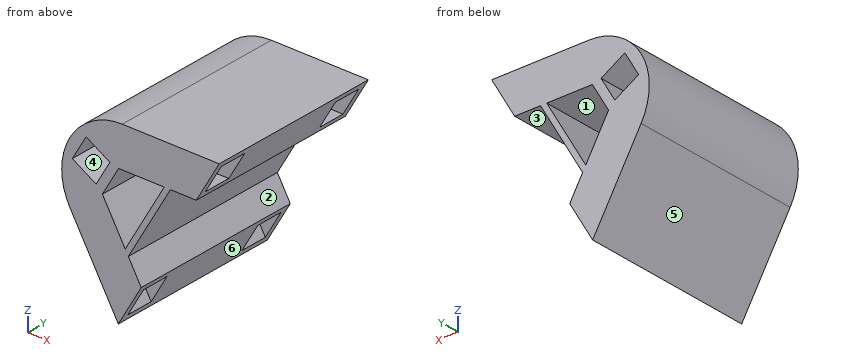
from build123d import *

# Parameters (mm, degrees)
BOSS_EXTRUDE1_DEPTH     = 130
SKETCH2_W               = 100.4
SKETCH2_H               = 20.4
CUT_EXTRUDE2_DEPTH      = 20.4
CUT_EXTRUDE3_DEPTH      = 238.223523286
FILLET1_R               = 45
CUT_EXTRUDE4_DEPTH      = 238.223523286
CUT_EXTRUDE4_DEPTH_BACK = 238.223523286
BOSS_EXTRUDE2_DEPTH     = 130


with BuildPart() as part:
    # Sketch1 → Boss-Extrude1 (new body)
    with BuildSketch(Plane(origin=(0, 0, 0), x_dir=(1, 0, 0), z_dir=(0, 1, 0))):
        Polygon((0, 0), (150, 0), (75, 129.903810568), align=None)
    extrude(amount=BOSS_EXTRUDE1_DEPTH)

    # Sketch2 → Cut-Extrude2 (cut)
    with BuildSketch(Plane(origin=(0, 5, 0), x_dir=(1, 0, 0), z_dir=(0, 1, 0))):
        Polygon((108.923840175, 138.261625339), (58.723840175, 51.312674799), (41.056921938, 61.512674799), (91.256921938, 148.461625339), align=None)
        with Locations((124, 15)):
            Rectangle(SKETCH2_W, SKETCH2_H)
    cut_extrude2 = extrude(amount=CUT_EXTRUDE2_DEPTH, mode=Mode.SUBTRACT)

    # Mirror1: Cut-Extrude2 across plane
    add(cut_extrude2.mirror(Plane.ZX.offset(65)), mode=Mode.SUBTRACT)

    # Sketch4 → Cut-Extrude3 (cut, through all)
    with BuildSketch(Plane(origin=(0, 0, 0), x_dir=(1, 0, 0), z_dir=(0, 1, 0))):
        Polygon((58.515583945, 45.561933634), (40.848665708, 35.361933634), (51.048665708, 17.695015397), (68.715583945, 27.895015397), align=None)
    extrude(amount=CUT_EXTRUDE3_DEPTH, mode=Mode.SUBTRACT)

    # Fillet1
    fillet1_edges = [part.edges().sort_by_distance(p)[0] for p in [
        (0, 65, 0),
    ]]
    fillet(fillet1_edges, radius=FILLET1_R)

    # Sketch27 → Cut-Extrude4 (cut, two sides: drawn at the far end of the back side and taken through both)
    with BuildSketch(Plane.XZ.offset(-CUT_EXTRUDE4_DEPTH_BACK)):
        Polygon((426.334426918, -29.530127019), (132.950773216, -29.530127019), (75.215746297, -29.530127019), (63.181713324, -50.373683549), (92.049226784, -100.373683549), (238.741053634, -354.45138071), (746.896447956, -647.835034411), (934.48982124, -322.913780721), align=None)
    extrude(amount=CUT_EXTRUDE4_DEPTH + CUT_EXTRUDE4_DEPTH_BACK, mode=Mode.SUBTRACT)

    # Sketch28 → Boss-Extrude2 (add)
    with BuildSketch(Plane.XZ):
        Polygon((109.106207099, -29.530127019), (80.126943725, -79.723683549), (82.436344802, -83.723683549), (113.725009252, -29.530127019), align=None)
    extrude(amount=-BOSS_EXTRUDE2_DEPTH)


solid = part.part
Can you work these out from the model? Positions are in its coordinate system, mm. Face numbers are marked on the shaded views. A direction names the side the tool comes from. Give positions to 0.01 mm unless a question says otherwise; leave off trailing zeros. Loops run counter-clockwise (first coordinate to the right, second up) from the corner with the lowest first, then second, coordinate; pieces in that order, holes last. Notation, with made-up numbers: (36.25, 54) -> (95.25, 54) arc R20 cw to (95.25, 65) -> close; hole circle Ø9 at (21, 10). An arc over 180 degrees is marked (long way). Use one line per item in the form item = value.
1) If we section it at C-C (z = -41): Please give me the cut outline in (x, y).
Answers:
outline = (33.12, 0) -> (50.61, 0) -> (50.61, 130) -> (33.12, 130) -> close; (61.15, 0) -> (68.59, 0) -> (68.59, 130) -> (61.15, 130) -> close; (102.48, 0) -> (107.1, 0) -> (107.1, 130) -> (102.48, 130) -> close
2) I need wall thicknesses on line 1 along Y through (x, z) = (122, -8.5); line 2 along Z through (x, y) = (92, 53); line 3 along Z through (x, y) = (83, 17.5). Which ranges of each line are inside material? Lowest first, please.
Answers:
line_1 = 0 to 5, 25.4 to 104.6, 125 to 130
line_2 = -100.46 to -100.29, -67.16 to -59.16, -29.53 to 0
line_3 = -93.36 to -84.7, -82.75 to -74.75, -29.53 to -25.2, -4.8 to 0
3) We'd pull the mould along X, two halves only. Please class the marked faces 4, 5 and 6: released by +X, released by -X, zero draft, split by the parting line, or undercut.
Answers:
face_4 = undercut
face_5 = released by -X
face_6 = released by +X
4) For the marked faces 1, 2 and 3, which set-ups out of +Z, -Z, +X, -X, +Y, -Y let a thin tool reach every point of the face, with its end or its side?
Answers:
face_1 = +Y, -Y
face_2 = +X, +Y, -Y
face_3 = -Z, +X, +Y, -Y
5) If we section it at B-B (x = 120.5): Please give me the cut outline in (y, z).
Answers:
outline = (0, -29.53) -> (130, -29.53) -> (130, 0) -> (0, 0) -> close; hole (5, -25.2) -> (25.4, -25.2) -> (25.4, -4.8) -> (5, -4.8) -> close; hole (104.6, -25.2) -> (125, -25.2) -> (125, -4.8) -> (104.6, -4.8) -> close
6) If we section it at A-A (y = 31): Please give me the cut outline in (x, z) (3 decimals), plus the area to 3 significant figures.
Answers:
outline = (38.971, -67.5) -> (75, -129.904) -> (92.049, -100.374) -> (82.436, -83.724) -> (113.725, -29.53) -> (132.951, -29.53) -> (150, 0) -> (77.942, 0) arc R45 ccw to start; hole (40.849, -35.362) -> (58.516, -45.562) -> (68.716, -27.895) -> (51.049, -17.695) -> close; hole (63.182, -50.374) -> (80.127, -79.724) -> (109.106, -29.53) -> (75.216, -29.53) -> close
area = 5,530 mm²
7) Will these pins go through, and if not, where does the flat tip stop? pin 1 (1.5 mm diameter, centred on x = 81, y = 65, fed in from -Z); pin 2 (10 mm diameter, centred on y = 19, z = -11.5, fed in from +X); pin 3 (10 mm diameter, centred on x = 95, y = 49, fed in from -Z).
Answers:
pin_1 = -120.81
pin_2 = 73.8
pin_3 = -103.92
8) If we section it at D-D (x = 104): Please give me the cut outline in (y, z), plus the area to 3 significant figures.
Answers:
outline = (0, -46.37) -> (130, -46.37) -> (130, -38.37) -> (0, -38.37) -> close; (0, -29.53) -> (130, -29.53) -> (130, 0) -> (0, 0) -> close; hole (5, -25.2) -> (25.4, -25.2) -> (25.4, -4.8) -> (5, -4.8) -> close; hole (104.6, -25.2) -> (125, -25.2) -> (125, -4.8) -> (104.6, -4.8) -> close
area = 4,050 mm²
